The model under review builds one solid part; all positions refer to its coordinate system, in mm. Coordinates: 2 decimals unless noted, no trailing zeros. Order: outer loops, then holes, each group sorted by start corner. A loop starts at its lowest first (then second) coordinate and runs counter-clockwise, first axis right, second up. Notation, with made-up numbers: M 25.5,-35.75 L 69.5,-35.75 A34 cw 69.5,-4.75 Z; hole C 62,-33.5 d10. An arc over 180 degrees is marked long. One line per item, written item: value.
```python
from build123d import *

# Parameters (mm, degrees)
BOX010_W         = 45
BOX010_H         = 15
BOX010_DEPTH     = 1
BOX013_W         = 9
BOX013_H         = 45
BOX013_DEPTH     = 1
ARRAY004_Y_COUNT = 4
ARRAY004_Y_PITCH = 90
BOX014_W         = 1
BOX014_H         = 45
BOX014_DEPTH     = 1
ARRAY003_Y_COUNT = 4
ARRAY003_Y_PITCH = 90
BOX016_W         = 125
BOX016_H         = 360
BOX016_DEPTH     = 1


with BuildPart() as box010:
    # Box010 → Box010 (new body)
    with BuildSketch(Plane(origin=(-80, 345, 0), x_dir=(1, 0, 0), z_dir=(0, 0, 1))):
        with Locations((22.5, 7.5)):
            Rectangle(BOX010_W, BOX010_H)
    extrude(amount=BOX010_DEPTH)


with BuildPart() as array004:
    # Box013 → Box013 (new body)
    with BuildSketch(Plane(origin=(-125, 0, 0), x_dir=(1, 0, 0), z_dir=(0, 0, 1))):
        with Locations((4.5, 22.5)):
            Rectangle(BOX013_W, BOX013_H)
    extrude(amount=BOX013_DEPTH)

    # Array004 Y: Array004 ×4


with BuildPart() as array004_1:
    add(array004.part)
    with Locations(*[(0, i * ARRAY004_Y_PITCH, 0) for i in range(1, ARRAY004_Y_COUNT)]):
        add(array004.part)


with BuildPart() as array004_2:
    # Array004 placement: moved
    add(array004_1.part.moved(Location((0, 22.5, 0))))


with BuildPart() as array003:
    # Box014 → Box014 (new body)
    with BuildSketch(Plane(origin=(-1, 0, 0), x_dir=(1, 0, 0), z_dir=(0, 0, 1))):
        with Locations((0.5, 22.5)):
            Rectangle(BOX014_W, BOX014_H)
    extrude(amount=BOX014_DEPTH)

    # Array003 Y: Array003 ×4


with BuildPart() as array003_1:
    add(array003.part)
    with Locations(*[(0, i * ARRAY003_Y_PITCH, 0) for i in range(1, ARRAY003_Y_COUNT)]):
        add(array003.part)


with BuildPart() as array003_2:
    # Array003 placement: moved
    add(array003_1.part.moved(Location((0, 22.5, 0))))


with BuildPart() as cut002008005:
    # Box016 → Box016 (new body)
    with BuildSketch(Plane(origin=(-125, 0, 0), x_dir=(1, 0, 0), z_dir=(0, 0, 1))):
        with Locations((62.5, 180)):
            Rectangle(BOX016_W, BOX016_H)
    extrude(amount=BOX016_DEPTH)

    # Cut002008003: cut Array003
    add(array003_2.part, mode=Mode.SUBTRACT)

    # Cut002008004: cut Array004
    add(array004_2.part, mode=Mode.SUBTRACT)

    # Cut002008005: cut Box010
    add(box010.part, mode=Mode.SUBTRACT)


solid = cut002008005.part
```
(1) We need section B-B, the plane y = 212.5. State the section outline as (x, z) points, plus the area to 3 significant figures.
Geometry results:
outline: M -116,0 L -1,0 L -1,1 L -116,1 Z
area: 115 mm2
(2) Insertion check: pin 1 Ø0.5 at (y, z) = (37.5, 0.5) entering from +X; pin 2 Ø0.5 at (y, z) = (43, 0.5) entering from -X. Each pin has a flat end and moves straight along its axis. Give the tip position at first contact, or say it passes through.
Geometry results:
pin 1: stops at x = -1
pin 2: stops at x = -116
(3) For L1, parallel to Y at x = -119.5, z = 0.8; L2, parallel to X at y = 226, z = 0.9; L3, parallel to Y at x = -38.5, z = 0.15, list the stretches that pass through material, from the lowest coordinate up.
Geometry results:
L1: y = 0 to 22.5, 67.5 to 112.5, 157.5 to 202.5, 247.5 to 292.5, 337.5 to 360
L2: x = -116 to -1
L3: y = 0 to 345
(4) We need section A-A, the plane x = -56. State the section outline as (y, z) points, plus the area to 3 significant figures.
Geometry results:
outline: M 0,0 L 345,0 L 345,1 L 0,1 Z
area: 345 mm2
